```python
from build123d import *

# Parameters (mm, degrees)
SKETCH_1_W          = 40
SKETCH_1_H          = 8
EXTRUDE_1_DEPTH     = 2
CUT_EXTRUDE_1_REACH = 22.494
SKETCH_2_R          = 2
CUT_EXTRUDE_2_REACH = 22.494
SKETCH_3_R          = 1.6
SKETCH_4_W          = 3
SKETCH_4_H          = 8
EXTRUDE_2_DEPTH     = 6
EXTRUDE_START       = 2
SKETCH_5_W          = 40
SKETCH_5_H          = 8
SKETCH_5_R          = 1.6
SKETCH_5_R_2        = 2
EXTRUDE_3_DEPTH     = 2
FILLET_1_R          = 2


with BuildPart() as part:
    # 草图1 → 凸台-拉伸1 (new body)
    with BuildSketch(Plane(origin=(0, 0, 0), x_dir=(1, 0, 0), z_dir=(0, 1, 0))):
        Rectangle(SKETCH_1_W, SKETCH_1_H)
    extrude(amount=EXTRUDE_1_DEPTH)

    # 草图2 → 切除-拉伸1 (cut, up to next)
    with BuildSketch(Plane(origin=(0, 2, 0), x_dir=(1, 0, 0), z_dir=(0, 1, 0)), mode=Mode.PRIVATE) as cut_extrude_1_sk1:
        with Locations(Location((0, 0, 0), (0, 0, 270))):
            Circle(SKETCH_2_R)
    cut_extrude_1_tool1 = extrude(cut_extrude_1_sk1.sketch, amount=-CUT_EXTRUDE_1_REACH, mode=Mode.PRIVATE) & part.part
    add(cut_extrude_1_tool1.solids().sort_by_distance((0, 2, 0))[0], mode=Mode.SUBTRACT)

    # 草图3 → 切除-拉伸2 (cut, up to next)
    with BuildSketch(Plane(origin=(0, 2, 0), x_dir=(1, 0, 0), z_dir=(0, 1, 0)), mode=Mode.PRIVATE) as cut_extrude_2_sk1:
        with Locations(Location((15, 0, 0), (0, 0, 270))):
            Circle(SKETCH_3_R)
    cut_extrude_2_tool1 = extrude(cut_extrude_2_sk1.sketch, amount=-CUT_EXTRUDE_2_REACH, mode=Mode.PRIVATE) & part.part
    # 草图3 → 切除-拉伸2 (cut, up to next)
    with BuildSketch(Plane(origin=(0, 2, 0), x_dir=(1, 0, 0), z_dir=(0, 1, 0)), mode=Mode.PRIVATE) as cut_extrude_2_sk2:
        with Locations(Location((-15, 0, 0), (0, 0, 90))):
            Circle(SKETCH_3_R)
    cut_extrude_2_tool2 = extrude(cut_extrude_2_sk2.sketch, amount=-CUT_EXTRUDE_2_REACH, mode=Mode.PRIVATE) & part.part
    add(cut_extrude_2_tool1.solids().sort_by_distance((15, 2, 0))[0], mode=Mode.SUBTRACT)
    add(cut_extrude_2_tool2.solids().sort_by_distance((-15, 2, 0))[0], mode=Mode.SUBTRACT)

    # 草图4 → 凸台-拉伸2 (add)
    with BuildSketch(Plane(origin=(0, 2, 0), x_dir=(1, 0, 0), z_dir=(0, 1, 0))):
        with Locations((-6, 0)):
            Rectangle(SKETCH_4_W, SKETCH_4_H)
        with Locations((6, 0)):
            Rectangle(SKETCH_4_W, SKETCH_4_H)
    extrude(amount=EXTRUDE_2_DEPTH)

    # 草图5 → 凸台-拉伸3 (add)
    with BuildSketch(Plane(origin=(0, 8, 0), x_dir=(1, 0, 0), z_dir=(0, 1, 0)).offset(EXTRUDE_START)):
        Rectangle(SKETCH_5_W, SKETCH_5_H)
        with Locations(Location((15, 0, 0), (0, 0, 270))):
            Circle(SKETCH_5_R, mode=Mode.SUBTRACT)
        with Locations(Location((0, 0, 0), (0, 0, 270))):
            Circle(SKETCH_5_R_2, mode=Mode.SUBTRACT)
        with Locations(Location((-15, 0, 0), (0, 0, 90))):
            Circle(SKETCH_5_R, mode=Mode.SUBTRACT)
    extrude(amount=-EXTRUDE_3_DEPTH)

    # 圆角1
    fillet_1_edges = [part.edges().sort_by_distance(p)[0] for p in [
        (20, 9, 4),
        (20, 9, -4),
        (-20, 9, -4),
        (-20, 9, 4),
        (20, 1, 4),
        (-20, 1, 4),
        (-20, 1, -4),
        (20, 1, -4),
    ]]
    fillet(fillet_1_edges, radius=FILLET_1_R)


solid = part.part
```
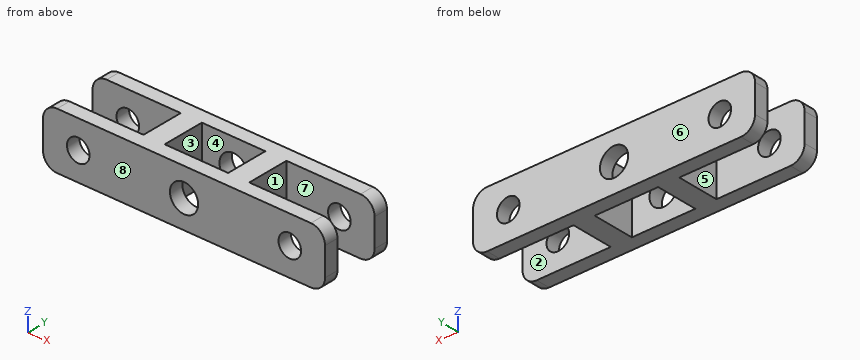
Read the model definition and answer for the solid it produces. Units are mm, in the model's axes. Face numbers are marked on the shaded views. A direction names the side the tool comes from. Coordinates: 2 decimals unless noted, no trailing zeros. Write each loop counter-clockwise with the first axis right and the second up, starting at its lowest first coordinate (ties: lowest second). Pieces come first, ordered by that corner, then holes. Notation, with made-up numbers: (51.5, 66) - (68.5, 66) arc R16 ccw to (68.5, 70) - close; hole circle Ø10 at (20.5, 32.5). An arc over 180 degrees is marked (long way). Answer as a JSON object with one key per item and string values. Group by question number.
1. The mould has two halves that part along X. Classify the marked faces 1, 2 and 3: +X half, -X half, draft (parallel to the pull), parting line (faces both ways), or undercut.
2. A cutting plane is placed at B-B (y = 6). Determine the outline of the cut face in (x, z).
3. A cutting plane is placed at C-C (z = 3.25). Determine the outline of the cut face in (x, y).
4. A cutting plane is placed at D-D (x = -15). Determine the outline of the cut face in (y, z), plus the area to 3 significant figures.
5. Consider L1, parallel to X at y = 1.15, z = 0; L2, parallel to X at y = 6.75, z = -2; L3, parallel to Z at x = -15, y = 1.1. Determine where each line is inside the solid, lowest interval first. Write a range as [from, to].
6. Which of the six approach directions +Z, -Z, +X, -X, +Y, -Y give full straight-line access (tool end or side, diameter ignored) to the marked faces 4, 5, 6, 7 and 8?
7. A cutting plane is placed at A-A (x = 0). Determine the outline of the cut face in (y, z), plus the area to 3 significant figures.
8. This flat-tipped pin is pushed along its axis until it touches: P1, Ø3, axis at y = 6, z = 2.5, coming from the -X side. Where does it stop, or does it pass through?
Worked out:
{
 "1": {"face 1": "+X half", "face 2": "draft", "face 3": "undercut"},
 "2": {"outline": "(-7.5, -4) - (-4.5, -4) - (-4.5, 4) - (-7.5, 4) - close; (4.5, -4) - (7.5, -4) - (7.5, 4) - (4.5, 4) - close"},
 "3": {"outline": "(-19.56, 0) - (19.56, 0) - (19.56, 2) - (7.5, 2) - (7.5, 8) - (19.56, 8) - (19.56, 10) - (-19.56, 10) - (-19.56, 8) - (-7.5, 8) - (-7.5, 2) - (-19.56, 2) - close; hole (-4.5, 2) - (4.5, 2) - (4.5, 8) - (-4.5, 8) - close"},
 "4": {"outline": "(0, -4) - (2, -4) - (2, -1.6) - (0, -1.6) - close; (0, 1.6) - (2, 1.6) - (2, 4) - (0, 4) - close; (8, -4) - (10, -4) - (10, -1.6) - (8, -1.6) - close; (8, 1.6) - (10, 1.6) - (10, 4) - (8, 4) - close", "area": "19.2 mm²"},
 "5": {"L1": "x = [-20, -16.6], [-13.4, -2], [2, 13.4], [16.6, 20]", "L2": "x = [-7.5, -4.5], [4.5, 7.5]", "L3": "z = [-4, -1.6], [1.6, 4]"},
 "6": {"face 4": "+Z, -Z", "face 5": "+Z, -Z, -X", "face 6": "+Z, -Z, +X, -X, +Y", "face 7": "+Z, -Z, +X", "face 8": "+Z, -Z, +X, -X, -Y"},
 "7": {"outline": "(0, -4) - (2, -4) - (2, -2) - (0, -2) - close; (0, 2) - (2, 2) - (2, 4) - (0, 4) - close; (8, -4) - (10, -4) - (10, -2) - (8, -2) - close; (8, 2) - (10, 2) - (10, 4) - (8, 4) - close", "area": "16.0 mm²"},
 "8": {"P1": "stops at x = -7.5"}
}
